```python
from build123d import *

# Parameters (mm, degrees)
BOSS_EXTRUDE1_DEPTH = 6.4
SKETCH2_R           = 1.5
CUT_EXTRUDE1_DEPTH  = 2
SKETCH3_R           = 1.5
CUT_EXTRUDE2_DEPTH  = 2
CHAMFER9_SIZE       = 1.5
CHAMFER10_SIZE      = 1.5
CHAMFER11_SIZE      = 1.5


with BuildPart() as part:
    # Sketch1 → Boss-Extrude1 (new body)
    with BuildSketch(Plane.XY):
        Polygon((-4.828427125, -2), (-2, -4.828427125), (-2, -30), (0, -30), (0, -2), (0, 0), (-30, 0), (-30, -2), align=None)
    extrude(amount=BOSS_EXTRUDE1_DEPTH)

    # Sketch2 → Cut-Extrude1 (cut)
    with BuildSketch(Plane(origin=(0, 0, 0), x_dir=(1, 0, 0), z_dir=(0, 1, 0))):
        with Locations((-23, -3.2)):
            Circle(SKETCH2_R)
        with Locations((-11, -3.2)):
            Circle(SKETCH2_R)
    extrude(amount=-CUT_EXTRUDE1_DEPTH, mode=Mode.SUBTRACT)

    # Sketch3 → Cut-Extrude2 (cut)
    with BuildSketch(Plane(origin=(0, 0, 0), x_dir=(0, 0, -1), z_dir=(1, 0, 0))):
        with Locations((-3.2, -11.193683163)):
            Circle(SKETCH3_R)
        with Locations((-3.2, -23.193683163)):
            Circle(SKETCH3_R)
    extrude(amount=-CUT_EXTRUDE2_DEPTH, mode=Mode.SUBTRACT)

    # Chamfer9
    chamfer9_edges = [part.edges().sort_by_distance(p)[0] for p in [
        (-17.414213562, -2, 0),
    ]]
    chamfer(chamfer9_edges, length=CHAMFER9_SIZE)

    # Chamfer10
    chamfer10_edges = [part.edges().sort_by_distance(p)[0] for p in [
        (-2, -17.414213562, 0),
        (-3.414213562, -3.414213562, 0),
    ]]
    chamfer(chamfer10_edges, length=CHAMFER10_SIZE)

    # Chamfer11
    chamfer11_edges = [part.edges().sort_by_distance(p)[0] for p in [
        (-17.414213562, -2, 6.4),
        (-3.414213562, -3.414213562, 6.4),
        (-2, -17.414213562, 6.4),
    ]]
    chamfer(chamfer11_edges, length=CHAMFER11_SIZE)


solid = part.part
```
The listing builds one solid part. Answer for the finished solid, in the listing's coordinates (mm). A direction names the side the tool comes from. Coordinates: 2 decimals unless noted, no trailing zeros. Write each loop counter-clockwise with the first axis right and the second up, starting at its lowest first coordinate (ties: lowest second). Pieces come first, ordered by that corner, then holes. Notation, with made-up numbers: M -24.5,-7 L 18.5,-7 A31 cw 18.5,31 Z; hole C 24,0 d10. An arc over 180 degrees is marked long. Use a Markdown table: item, result. Add a question column.
1. Section A-A (x = -23) is taken. Give the vertices of the cut face in (y, z), plus the area to 3 significant figures.
2. Straight lines are drawn through the part: line 1 along Y through (x, z) = (-1.2, 3.2); line 2 along X through (y, z) = (-1.3, 3.2); line 3 along Y through (x, z) = (-1.25, 2.75). For each, find the intervals that lie inside material, in ascending order. Write a range as [from, to].
3. Section B-B (y = -12) is taken. Give the vertices of the cut face in (x, z).
4. Which of the six approach directions +Z, -Z, +X, -X, +Y, -Y give full straight-line access (tool end or side, diameter ignored) to faces 5 (the flat face through (-17.3, -1.2, 0.7)), 6 (the cylindrical face through (-24.5, -0.99, 3.13)), 7 (the flat face through (-17.3, -1.2, 5.7)), 8 (the flat face through (-1, -30, 3)), 9 (the flat face through (-2, -17, 3))?
5. Given P1, Ø1.8, axis at x = -11, z = 3.2, coming from the -Y side; P2, Ø1, axis at x = -15.5, z = 3.5, coming from the -Y side; P3, Ø1, axis at y = -21.5, z = 3.5, coming from the -X side, each flat-ended and moving along its own axis, determine where each tip first touches the part or whether it passes through.
6. For a pull along Y with two mould halves and no side action, classify faces 1 (the flat face through (-18, -2, 3)), 2 (the flat face through (-1.3, -16.9, 0.8)), 3 (the cylindrical face through (-0.986, -24.658, 3.525)), 4 (the cylindrical face through (-0.99, -12.11, 4.39)) as +Y half, -Y half, draft (parallel to the pull), parting line (faces both ways), or undercut.
7. Section C-C (x = -6) is taken. Give the vertices of the cut face in (y, z).
Data:
| question | item | result |
|---|---|---|
| 1 | outline | M -2,1.5 L -0.5,0 L 0,0 L 0,1.7 L -2,1.7 Z; M -2,4.7 L 0,4.7 L 0,6.4 L -0.5,6.4 L -2,4.9 Z |
| 1 | area | 4.55 mm2 |
| 2 | line 1 | y = [-30, -24.69], [-21.69, -12.69], [-9.69, 0] |
| 2 | line 2 | x = [-30, -24.5], [-21.5, -12.5], [-9.5, 0] |
| 2 | line 3 | y = [-30, -24.62], [-21.76, -12.62], [-9.76, 0] |
| 3 | outline | M -2,1.5 L -0.5,0 L 0,0 L 0,1.94 L -2,1.94 Z; M -2,4.46 L 0,4.46 L 0,6.4 L -0.5,6.4 L -2,4.9 Z |
| 4 | face 5 | -Z, -X, -Y |
| 4 | face 6 | +Y, -Y |
| 4 | face 7 | +Z, -X, -Y |
| 4 | face 8 | +Z, -Z, +X, -X, -Y |
| 4 | face 9 | +Z, -Z, -X, -Y |
| 5 | P1 | passes through |
| 5 | P2 | stops at y = -2 |
| 5 | P3 | stops at x = -2 |
| 6 | face 1 | -Y half |
| 6 | face 2 | draft |
| 6 | face 3 | undercut |
| 6 | face 4 | undercut |
| 7 | outline | M -2,1.5 L -0.5,0 L 0,0 L 0,6.4 L -0.5,6.4 L -2,4.9 Z |
